Build history of the part. All positions in model axes, mm. A direction names the side the tool comes from. Give positions to 0.01 mm unless a question says otherwise; leave off trailing zeros. Order: outer loops, then holes, each group sorted by start corner. A loop starts at its lowest first (then second) coordinate and runs counter-clockwise, first axis right, second up. Notation, with made-up numbers: (-27, -24.75) - (-10, -24.75) arc R11 ccw to (-10, -15.75) - close; hole circle Ø3 at (45, 85.5). An arc over 180 degrees is marked (long way). One line per item, written item: value.
Autodesk Inventor part; units mm, degrees
ref_plane "YZ Plane" through (0, 0, 0) normal (1, 0, 0) x (0, 1, 0)
ref_plane "XZ Plane" through (0, 0, 0) normal (0, 1, 0) x (-1, 0, 0)
ref_plane "XY Plane" through (0, 0, 0) normal (0, 0, 1) x (1, 0, 0)
sketch "Sketch1" plane through (0, 0, 0) normal (1, 0, 0) x (0, 1, 0)
  circle A0 centre (0, 0) radius 20
  dimension "d0" = 40
extrude "Extrusion1" add sketch "Sketch1" along normal mid plane 106
sketch "Sketch2" plane through (53, 0, 0) normal (1, 0, 0) x (0, 0, -1)
  circle A0 centre (0, 0) radius 10
  dimension "d3" = 20
extrude "Extrusion2" cut sketch "Sketch2" against normal blind 10
sketch "Sketch3" plane through (-53, 0, 0) normal (-1, 0, 0) x (0, 0, 1)
  circle A0 centre (0, 0) radius 10
  dimension "d6" = 20
extrude "Extrusion3" cut sketch "Sketch3" against normal blind 10
sketch "Sketch5" plane through (0, 0, 0) normal (0, 0, 1) x (1, 0, 0)
  circle A0 centre (0, 0) radius 20
  line L0 (-53, 20) -> (53, 20)
extrude "Extrusion4" add sketch "Sketch5" along normal mid plane 145
sketch "Sketch6" plane through (0, 0, 72.5) normal (0, 0, 1) x (1, 0, 0)
  circle A0 centre (0, 0) radius 5
  dimension "d12" = 10
extrude "Extrusion5" add sketch "Sketch6" along normal blind 10
sketch "Sketch7" plane through (0, 0, -72.5) normal (0, 0, -1) x (-1, 0, 0)
  circle A0 centre (0, 0) radius 5
extrude "Extrusion6" add sketch "Sketch7" along normal blind 10
properties part number "AERO - Arm"
(1) Slice it at B-B, the plane x = -13. Give the cut face in (y, z), and give its area (3 significant figures).
Completed:
outline: (-15.2, -72.5) - (15.2, -72.5) - (15.2, -13) arc R20 ccw to (15.2, 13) - (15.2, 72.5) - (-15.2, 72.5) - (-15.2, 13) arc R20 ccw to (-15.2, -13) - close
area: 4,580 mm²
(2) Slice it at D-D, the plane y = -12.5. Give the cut face in (x, z).
Completed:
outline: (-53, -15.61) - (-15.61, -15.61) - (-15.61, -72.5) - (15.61, -72.5) - (15.61, -15.61) - (53, -15.61) - (53, 15.61) - (15.61, 15.61) - (15.61, 72.5) - (-15.61, 72.5) - (-15.61, 15.61) - (-53, 15.61) - close
(3) Drill centre lines: line 1 (Y direction, x = -48.5, z = 0); line 2 (X direction, y = -9.5, z = -1.5); line 3 (Z direction, x = 8.5, y = 14.5). Where is each one in solid material? Low to high.
Completed:
line 1: -20 to -10, 10 to 20
line 2: -43 to 43
line 3: -72.5 to 72.5
(4) Slice it at A-A, the plane y = 0. Give the cut face in (x, z).
Completed:
outline: (-53, -20) - (-20, -20) - (-20, -72.5) - (-5, -72.5) - (-5, -82.5) - (5, -82.5) - (5, -72.5) - (20, -72.5) - (20, -20) - (53, -20) - (53, -10) - (43, -10) - (43, 10) - (53, 10) - (53, 20) - (20, 20) - (20, 72.5) - (5, 72.5) - (5, 82.5) - (-5, 82.5) - (-5, 72.5) - (-20, 72.5) - (-20, 20) - (-53, 20) - (-53, 10) - (-43, 10) - (-43, -10) - (-53, -10) - close
(5) Pin check, flat tips, straight feed: P1, Ø12, axis at x = -24, y = -1, coming from the -Z side; P2, Ø4, axis at y = -10.5, z = -40.5, coming from the -X side; P3, Ø3, axis at x = -13, z = -30.5, coming from the +Y side. Stop position of each tip, or through.
Completed:
P1: z = -72.5
P2: x = -18.1
P3: y = 16.36
(6) Slice it at C-C, the plane z = -4.5. Give the cut face in (x, y).
Completed:
outline: (-53, -19.49) - (-4.5, -19.49) arc R20 ccw to (4.5, -19.49) - (53, -19.49) - (53, -8.93) - (43, -8.93) - (43, 8.93) - (53, 8.93) - (53, 19.49) - (4.5, 19.49) arc R20 ccw to (-4.5, 19.49) - (-53, 19.49) - (-53, 8.93) - (-43, 8.93) - (-43, -8.93) - (-53, -8.93) - close
(7) 3-axis set-ups, long thin cutter, end or side, ignore diameter. For faces 4 (the face through (32.02, -19.98, -0.88)), 5 (the face through (19.076, -6.007, 43.798)), 6 (the face through (1.08, 4.88, -77.43)): which of +Z, -Z, +X, -X, +Y, -Y reach the whole face in a straight line?
Completed:
face 4: +X
face 5: +Z
face 6: -Z
(8) Pull direction Y, two halves, no side cores. Call faces 1 (the face through (53, -5, 9)), 2 (the face through (48.07, -9.76, 2.17)), 3 (the face through (19.076, 6.007, -43.798)): +Y half, -Y half, draft (parallel to the pull), parting line (faces both ways), or undercut.
Completed:
face 1: draft
face 2: undercut
face 3: parting line
